from build123d import *

# Parameters (mm, degrees)
SKETCH1_R           = 4
SKETCH1_W           = 4.1
SKETCH1_H           = 15
SKETCH1_W_2         = 15
SKETCH1_H_2         = 4.1
SKETCH1_W_3         = 12
SKETCH1_H_3         = 28
SKETCH1_W_4         = 28
SKETCH1_H_4         = 12
BOSS_EXTRUDE1_DEPTH = 4.1
FILLET4_R           = 10


with BuildPart() as part:
    # Sketch1 → Boss-Extrude1 (new body)
    with BuildSketch(Plane(origin=(0, 0, 0), x_dir=(1, 0, 0), z_dir=(0, 1, 0))):
        Polygon((-25, 67), (-67, 25), (-80, 25), (-80, -25), (-67, -25), (-25, -67), (-25, -80), (25, -80), (25, -67), (67, -25), (80, -25), (80, 25), (67, 25), (25, 67), (25, 80), (-25, 80), align=None)
        with Locations((-38.183766184, -38.183766184)):
            Circle(SKETCH1_R, mode=Mode.SUBTRACT)
        with Locations((-22.95, 37.5)):
            Rectangle(SKETCH1_W, SKETCH1_H, mode=Mode.SUBTRACT)
        with Locations((-37.5, 22.95)):
            Rectangle(SKETCH1_W_2, SKETCH1_H_2, mode=Mode.SUBTRACT)
        with Locations((37.5, -22.95)):
            Rectangle(SKETCH1_W_2, SKETCH1_H_2, mode=Mode.SUBTRACT)
        with Locations((22.95, -37.5)):
            Rectangle(SKETCH1_W, SKETCH1_H, mode=Mode.SUBTRACT)
        with Locations((37.5, 22.95)):
            Rectangle(SKETCH1_W_2, SKETCH1_H_2, mode=Mode.SUBTRACT)
        with Locations((-37.5, -22.95)):
            Rectangle(SKETCH1_W_2, SKETCH1_H_2, mode=Mode.SUBTRACT)
        with Locations((22.95, 37.5)):
            Rectangle(SKETCH1_W, SKETCH1_H, mode=Mode.SUBTRACT)
        with Locations((-22.95, -37.5)):
            Rectangle(SKETCH1_W, SKETCH1_H, mode=Mode.SUBTRACT)
        Polygon((-36.062445841, 4.949747468), (-25.455844123, -5.656854249), (-28.354981926, -8.555992052), (-38.961583643, 2.050609665), align=None, mode=Mode.SUBTRACT)
        Polygon((-8.555992052, -28.354981926), (2.050609665, -38.961583643), (4.949747468, -36.062445841), (-5.656854249, -25.455844123), align=None, mode=Mode.SUBTRACT)
        with Locations((-61, 0)):
            Rectangle(SKETCH1_W_3, SKETCH1_H_3, mode=Mode.SUBTRACT)
        with Locations((61, 0)):
            Rectangle(SKETCH1_W_3, SKETCH1_H_3, mode=Mode.SUBTRACT)
        with Locations((0, 61)):
            Rectangle(SKETCH1_W_4, SKETCH1_H_4, mode=Mode.SUBTRACT)
        with Locations((0, -61)):
            Rectangle(SKETCH1_W_4, SKETCH1_H_4, mode=Mode.SUBTRACT)
        Polygon((38.961583643, -2.050609665), (36.062445841, -4.949747468), (25.455844123, 5.656854249), (28.354981926, 8.555992052), align=None, mode=Mode.SUBTRACT)
        Polygon((8.555992052, 28.354981926), (-2.050609665, 38.961583643), (-4.949747468, 36.062445841), (5.656854249, 25.455844123), align=None, mode=Mode.SUBTRACT)
    extrude(amount=BOSS_EXTRUDE1_DEPTH)

    # Fillet4
    fillet4_edges = [part.edges().sort_by_distance(p)[0] for p in [
        (-25, 2.05, 67),
        (-67, 2.05, -25),
        (-25, 2.05, -67),
        (25, 2.05, -67),
        (67, 2.05, 25),
    ]]
    fillet(fillet4_edges, radius=FILLET4_R)


solid = part.part
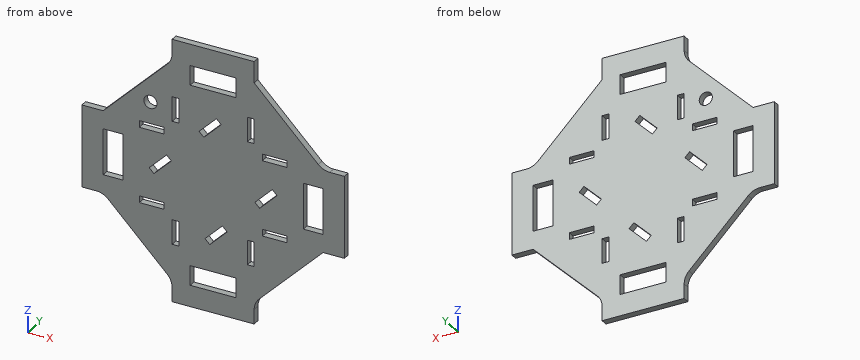
Source: CAD feature listing. Evaluate the final solid. Frame: model axes, mm. Give positions to 0.01 mm unless a question says otherwise; leave off trailing zeros. Order: outer loops, then holes, each group sorted by start corner. A loop starts at its lowest first (then second) coordinate and runs counter-clockwise, first axis right, second up. Notation, with made-up numbers: (0, 18.5) -> (53, 18.5) arc R19 ccw to (53, 55.5) -> close; hole circle Ø9 at (-5, 89.25). An arc over 180 degrees is marked (long way). Write item = value, one per line.
Item 1: Section query C-C (x = 23). Output: boundary loops of the cut face in (y, z).
Check result:
outline = (0, -80) -> (4.1, -80) -> (4.1, -45) -> (0, -45) -> close; (0, -30) -> (4.1, -30) -> (4.1, 30) -> (0, 30) -> close; (0, 45) -> (4.1, 45) -> (4.1, 80) -> (0, 80) -> close
Item 2: Contact query for flat-ended pins moving along their axis: pin 1 (1.2 mm diameter, centred on x = 37, y = 3, fed in from -Z); pin 2 (1.5 mm diameter, centred on x = -50.5, y = 2, fed in from -Z); pin 3 (2 mm diameter, centred on y = 2, z = -37.5, fed in from +X). Output: stop coordinate, or through.
Check result:
pin_1 = -55.6
pin_2 = -42.25
pin_3 = 55.5
Item 3: Section query D-D (y = 1.4). State how many separate pieces and enclosed holes the cut face has, then the cut area to 3 significant figures.
Check result:
separate_pieces = 1
enclosed_holes = 17
area = 14,900 mm²
Item 4: Section query B-B (z = -11). Output: boundary loops of the cut face in (x, y), then the cut area to 3 significant figures.
Check result:
outline = (-80, 0) -> (-67, 0) -> (-67, 4.1) -> (-80, 4.1) -> close; (-55, 0) -> (55, 0) -> (55, 4.1) -> (-55, 4.1) -> close; (67, 0) -> (80, 0) -> (80, 4.1) -> (67, 4.1) -> close
area = 558 mm²
Item 5: Section query A-A (x = 58.5). Output: boundary loops of the cut face in (y, z), then the cut area to 3 significant figures.
Check result:
outline = (0, -33.5) -> (4.1, -33.5) -> (4.1, -14) -> (0, -14) -> close; (0, 14) -> (4.1, 14) -> (4.1, 33.5) -> (0, 33.5) -> close
area = 160 mm²
Item 6: Ray query, probe 1 along Z at (x, y) = (22.5, 3.45); probe 2 along X at (y, z) = (1.45, -13.5); probe 3 along Z at (x, y) = (3.5, 0.3). Return the intervals inside material, ascending.
Check result:
probe_1 = -80 to -45, -30 to 30, 45 to 80
probe_2 = -80 to -67, -55 to 55, 67 to 80
probe_3 = -80 to -67, -55 to -33.41, -27.61 to 34.61, 37.51 to 55, 67 to 80
